from build123d import *

# Parameters (mm, degrees)
F1_R      = 19.907119
F2_DEPTH  = 12.7
F0_R      = 11.75258
F3_DEPTH  = 12.7
F4_W      = 25.4
F4_H      = 25.4
F5_DEPTH  = 12.7
F6_W      = 20.955
F6_H      = 10.16
F7_DEPTH  = 19.05
F8_R      = 1.075724
F9_DEPTH  = 5.715
F10_R     = 1.861497
F11_DEPTH = 19.05


with BuildPart() as f2:
    # F1 (on Top) → F2 (new body)
    with BuildSketch(Plane.XY):
        Circle(F1_R)
    extrude(amount=-F2_DEPTH)

    # F0 (on Top) → F3 (cut)
    with BuildSketch(Plane.XY):
        Circle(F0_R)
    extrude(amount=-F3_DEPTH, mode=Mode.SUBTRACT)

    # F4 (on Top) → F5 (join)
    with BuildSketch(Plane.XY):
        Rectangle(F4_W, F4_H)
    extrude(amount=F5_DEPTH)

    # F6 (on Top) → F7 (join)
    with BuildSketch(Plane.XY):
        Rectangle(F6_W, F6_H)
    extrude(amount=F7_DEPTH)

    # F8 (on Front) → F9 (cut, symmetric)
    with BuildSketch(Plane.XZ):
        with Locations((0, 17.094158)):
            Circle(F8_R)
    extrude(amount=F9_DEPTH, both=True, mode=Mode.SUBTRACT)

    # F10 (on Top) → F11 (cut)
    with BuildSketch(Plane.XY):
        Circle(F10_R)
    extrude(amount=F11_DEPTH, mode=Mode.SUBTRACT)


solid = f2.part
Can you work these out from the model? Positions are in its coordinate system, mm. A direction names the side the tool comes from. Round coordinates to 2 decimals unless told otherwise and drop trailing zeros. Order: outer loops, then holes, each group sorted by start corner. A loop starts at its lowest first (then second) coordinate and runs counter-clockwise, first axis right, second up. Notation, with made-up numbers: M -39.5,47 L -22.5,47 A25 ccw -22.5,61 Z; hole C -24,2.25 d7. An arc over 180 degrees is marked long. Use a Markdown table: item, result.
1) Imagine slicing it at D-D (x = -7). List the corners of the cut face in (y, z) for me.
Geometry says:
| item | result |
|---|---|
| outline | M -18.64,-12.7 L -9.44,-12.7 L -9.44,0 L 9.44,0 L 9.44,-12.7 L 18.64,-12.7 L 18.64,0 L 12.7,0 L 12.7,12.7 L 5.08,12.7 L 5.08,19.05 L -5.08,19.05 L -5.08,12.7 L -12.7,12.7 L -12.7,0 L -18.64,0 Z |
2) If I drill on line 1 along Y through (x, z) = (0, 10); line 2 along Y through (x, z) = (0, -4.25); line 3 along X through (y, z) = (3, 5.5), over which ranges is the centre line in solid material (lowest first)?
Geometry says:
| item | result |
|---|---|
| line 1 | y = -12.7 to -1.86, 1.86 to 12.7 |
| line 2 | y = -19.91 to -11.75, 11.75 to 19.91 |
| line 3 | x = -12.7 to 12.7 |
3) Imagine slicing it at B-B (y = 0). List the corners of the cut face in (x, z) for me, then the cut area to 3 significant figures.
Geometry says:
| item | result |
|---|---|
| outline | M -19.91,-12.7 L -11.75,-12.7 L -11.75,0 L -1.86,0 L -1.86,19.05 L -10.48,19.05 L -10.48,12.7 L -12.7,12.7 L -12.7,0 L -19.91,0 Z; M 1.86,0 L 11.75,0 L 11.75,-12.7 L 19.91,-12.7 L 19.91,0 L 12.7,0 L 12.7,12.7 L 10.48,12.7 L 10.48,19.05 L 1.86,19.05 Z |
| area | 592 mm² |
4) If we mould it in two halves opening along Y, with no side actions, what happens to faces 1 (the face through (10.478, 0, 16)), 2 (the face through (-0.1, -5.08, 15.8)), 3 (the face through (1.776, 0.559, 9.392))? For each: +Y half, -Y half, draft (parallel to the pull), parting line (faces both ways), or undercut.
Geometry says:
| item | result |
|---|---|
| face 1 | draft |
| face 2 | -Y half |
| face 3 | undercut |
5) I'm going to push flat-ended pins straight in: P1, Ø6.5, axis at y = -0.5, z = 7, coming from the -X side; P2, Ø6, axis at x = 6.5, y = -3, coming from the -Z side; P3, Ø2, axis at y = -10, z = 6.5, coming from the +X side; P4, Ø3, axis at x = 15.5, z = 9, coming from the +Y side. Where does each tip first touch, or does it pass through?
Geometry says:
| item | result |
|---|---|
| P1 | stops at x = -12.7 |
| P2 | stops at z = 0 |
| P3 | stops at x = 12.7 |
| P4 | passes through |
6) Imagine slicing it at A-A (x = 0). List the corners of the cut face in (y, z) for me.
Geometry says:
| item | result |
|---|---|
| outline | M -19.91,-12.7 L -11.75,-12.7 L -11.75,0 L -1.86,0 L -1.86,16.02 L -5.08,16.02 L -5.08,12.7 L -12.7,12.7 L -12.7,0 L -19.91,0 Z; M -5.08,18.17 L -1.86,18.17 L -1.86,19.05 L -5.08,19.05 Z; M 1.86,0 L 11.75,0 L 11.75,-12.7 L 19.91,-12.7 L 19.91,0 L 12.7,0 L 12.7,12.7 L 5.08,12.7 L 5.08,16.02 L 1.86,16.02 Z; M 1.86,18.17 L 5.08,18.17 L 5.08,19.05 L 1.86,19.05 Z |
7) On a 3-axis mill with a long thin cutter (end or side, diameter ignored), from which of +Z, -Z, +X, -X, +Y, -Y can I reach the whole of each face in a straight line? I mean faces 4 (the face through (12.7, 0, 6)), 5 (the face through (6.32, 9.91, -6.26)), 6 (the face through (-12.7, 0, 6)). Say none if no direction works.
Geometry says:
| item | result |
|---|---|
| face 4 | +Z, +X, +Y, -Y |
| face 5 | -Z |
| face 6 | +Z, -X, +Y, -Y |
8) Imagine slicing it at C-C (z = 5.5). List the corners of the cut face in (x, y) for me, then the cut area to 3 significant figures.
Geometry says:
| item | result |
|---|---|
| outline | M -12.7,-12.7 L 12.7,-12.7 L 12.7,12.7 L -12.7,12.7 Z; hole C 0,0 d3.72 |
| area | 634 mm² |
